CAD build for the part. Positions are in the model's coordinates, mm. Face numbers are marked on the shaded views. A direction names the side the tool comes from. Give positions to 0.01 mm unless a question says otherwise; leave off trailing zeros. Order: outer loops, then holes, each group sorted by start corner. A loop starts at its lowest first (then second) coordinate and runs counter-clockwise, first axis right, second up.
Item 1: Band-saw the part on A-A on x = 15. Give the cut face in (y, z), plus the area to 3 significant figures.
Item 2: Band-saw the part on C-C on y = -3. Give the cut face in (x, z).
Item 3: Two-plate mould, pull along X, no slides. Class the marked faces 6, 7, 8 and 9: released by +X, released by -X, zero draft, split by the parting line, or undercut.
Item 4: Which spindle directions (+Z, -Z, +X, -X, +Y, -Y) get a long thin tool onto all of the face, cutting with end or side? Do the marked faces 1, 2, 3, 4 and 5. Say none if no direction does.
Item 5: Wall check: L1, parallel to Y at x = -14.5, z = -7.5; L2, parallel to Y at x = 0, z = 5.25; L3, parallel to X at y = -1.75, z = 5.5. Give the ranges that are in metal, low to high.
Item 6: Flat gauge pins, fed straight in: P1, Ø8.5, axis at x = -15.5, z = 4, coming from the +Y side; P2, Ø2, axis at x = -5.5, z = -3.5, coming from the +Y side. Where does each tip first touch, or does it go through?
Item 7: Band-saw the part on B-B on z = 0.75. Give the cut face in (x, y).
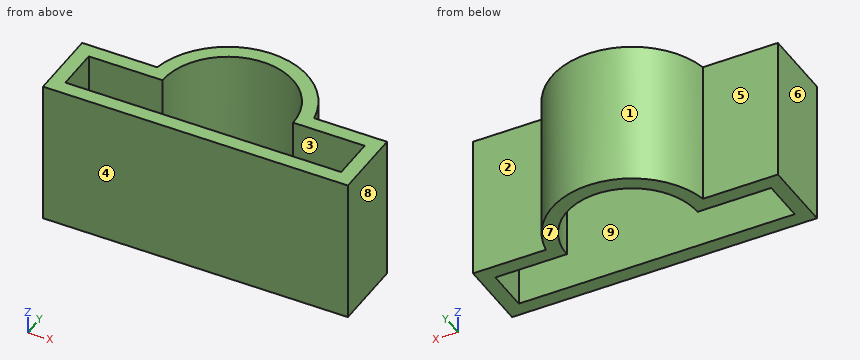
```python
from build123d import *

# Parameters (mm, degrees)
BOSS_EXTRUDE1_DEPTH = 10


with BuildPart() as part:
    # Sketch1 → Boss-Extrude1 (new, symmetric)
    with BuildSketch(Plane.XY):
        with BuildLine():
            Line((10.816653826, 2), (20.85239712, 2))
            Line((20.85239712, 2), (20.85239712, -8))
            Line((20.85239712, -8), (-21.14760288, -8))
            Line((-21.14760288, -8), (-21.14760288, 2))
            Line((-21.14760288, 2), (-10.816653826, 2))
            ThreePointArc((-10.816653826, 2), (0, 11), (10.816653826, 2))
        make_face()
        with BuildLine():
            Line((9, 0), (18.85239712, 0))
            Line((18.85239712, 0), (18.85239712, -6))
            Line((18.85239712, -6), (-19.14760288, -6))
            Line((-19.14760288, -6), (-19.14760288, 0))
            Line((-19.14760288, 0), (-9, 0))
            ThreePointArc((-9, 0), (0, 9), (9, 0))
        make_face(mode=Mode.SUBTRACT)
    extrude(amount=BOSS_EXTRUDE1_DEPTH, both=True)


solid = part.part
```
The answers:
1. outline: (-8, -10) - (-6, -10) - (-6, 10) - (-8, 10) - close; (0, -10) - (2, -10) - (2, 10) - (0, 10) - close
1. area: 80.0 mm2
2. outline: (-21.15, -10) - (-19.15, -10) - (-19.15, 10) - (-21.15, 10) - close; (18.85, -10) - (20.85, -10) - (20.85, 10) - (18.85, 10) - close
3. face 6: released by -X
3. face 7: zero draft
3. face 8: released by +X
3. face 9: undercut
4. face 1: +Z, -Z, +Y
4. face 2: +Z, -Z, +X, +Y
4. face 3: +Z, -Z
4. face 4: +Z, -Z, +X, -X, -Y
4. face 5: +Z, -Z, -X, +Y
5. L1: y = -8 to -6, 0 to 2
5. L2: y = -8 to -6, 9 to 11
5. L3: x = -21.15 to -19.15, 18.85 to 20.85
6. P1: stops at y = 2
6. P2: stops at y = 10.04
7. outline: (-21.15, -8) - (20.85, -8) - (20.85, 2) - (10.82, 2) arc R11 ccw to (-10.82, 2) - (-21.15, 2) - close; hole (-19.15, -6) - (18.85, -6) - (18.85, 0) - (9, 0) arc R9 ccw to (-9, 0) - (-19.15, 0) - close
